from build123d import *

# Parameters (mm, degrees)
BOSS_EXTRUDE1_DEPTH     = 19.05
SKETCH2_R               = 1.26619
CUT_EXTRUDE1_DEPTH      = 18.879441165
CUT_EXTRUDE1_DEPTH_BACK = 28.404441165
SKETCH3_R               = 1.26619
CUT_EXTRUDE2_DEPTH      = 4.175


with BuildPart() as part:
    # Sketch1 → Boss-Extrude1 (new body)
    with BuildSketch(Plane(origin=(0, 0, 0), x_dir=(1, 0, 0), z_dir=(0, 1, 0))):
        Polygon((0, -22.641941165), (0, 22.641941165), (3.175, 22.641941165), (3.175, 4.7625), (21.59, 4.7625), (21.59, 1.5875), (3.175, 1.5875), (3.175, -1.5875), (21.59, -1.5875), (21.59, -4.7625), (3.175, -4.7625), (3.175, -22.641941165), align=None)
    extrude(amount=BOSS_EXTRUDE1_DEPTH)

    # Sketch2 → Cut-Extrude1 (cut, two sides)
    with BuildSketch(Plane.XY.offset(4.7625)) as cut_extrude1_sk:
        with Locations((12.065, 9.525)):
            Circle(SKETCH2_R)
    extrude(amount=CUT_EXTRUDE1_DEPTH, mode=Mode.SUBTRACT)
    extrude(cut_extrude1_sk.sketch, amount=-CUT_EXTRUDE1_DEPTH_BACK, mode=Mode.SUBTRACT)

    # Sketch3 → Cut-Extrude2 (cut, through all)
    with BuildSketch(Plane(origin=(3.175, 0, 0), x_dir=(0, 0, -1), z_dir=(1, 0, 0))):
        with Locations((-15.021941165, 14.9225)):
            Circle(SKETCH3_R)
        with Locations((-15.021941165, 4.1275)):
            Circle(SKETCH3_R)
        with Locations((15.021941165, 4.1275)):
            Circle(SKETCH3_R)
        with Locations((15.021941165, 14.9225)):
            Circle(SKETCH3_R)
    extrude(amount=-CUT_EXTRUDE2_DEPTH, mode=Mode.SUBTRACT)


solid = part.part
Source: CAD feature listing. Evaluate the final solid. Frame: model axes, mm. A direction names the side the tool comes from. Coordinates: 2 decimals unless noted, no trailing zeros. Order: outer loops, then holes, each group sorted by start corner. A loop starts at its lowest first (then second) coordinate and runs counter-clockwise, first axis right, second up. Notation, with made-up numbers: M 76.5,-32 L 126.5,-32 A29 ccw 126.5,-12 Z; hole C -5.75,-22 d10. An arc over 180 degrees is marked long. Write each question's results on one line, items separated by ' | '. Start each with the question number.
Item 1: First-contact query: pin 1 Ø1.5 at (y, z) = (13.5, 7.5) entering from +X (3 decimals); pin 2 Ø4 at (x, y) = (12.065, 9.525) entering from +Z; pin 3 Ø2 at (y, z) = (14.92, -15.02) entering from +X; pin 4 Ø10 at (x, y) = (12, 6.5) entering from -Z. Flat tips, straight axial feed; report the tip coordinate or a pass-through.
Item 2: Cut plane A-A (x = 12). Return loops of the section in (y, z), and give its area (3 significant figures).
Item 3: Line query: probe 1 along Z at (x, y) = (6, 11.5); probe 2 along X at (y, z) = (7.5, -0.5) (3 decimals); probe 3 along Y at (x, z) = (11.25, 4.5). Output: solid intervals per line, ascending.
Item 4: Cut plane D-D (z = -18). Return loops of the section in (x, y) (3 decimals).
Item 5: Draft query along Y for faces 1 (the face through (14, 9, 1.588)), 2 (the face through (1.61, 14.15, -14.02)), 3 (the face through (5, 0, -2)), 4 (the face through (1.61, 4.183, -13.757)). Return one class per face: pulls with the +Y half, pulls with the -Y half, needs draft (parallel to the pull), parting line crosses it, or undercut.
Item 6: Cut plane C-C (y = 15.5). Return loops of the section in (x, z) (1 decimal), and give its area (3 significant figures).
Item 7: Cut plane B-B (x = 8.25). Return loops of the section in (y, z).
Item 8: Set-up query: faces 5 (the face through (10, 9, 4.762)), 6 (the face through (2, 9, 22.642)), 7 (the face through (13.27, 9.91, 3.2)), 8 (the face through (3.175, 9, 0)), 9 (the face through (3.175, 9, -14)). Return all of +Z, -Z, +X, -X, +Y, -Y with unobstructed straight access to the full face (end or side cutting, diameter ignored); none if empty.
Checked values:
1) pin 1: stops at x = 3.175 | pin 2: stops at z = 4.76 | pin 3: passes through | pin 4: stops at z = -4.76
2) outline: M 0,-4.76 L 8.26,-4.76 L 8.26,-1.59 L 0,-1.59 Z; M 0,1.59 L 8.26,1.59 L 8.26,4.76 L 0,4.76 Z; M 10.79,-4.76 L 19.05,-4.76 L 19.05,-1.59 L 10.79,-1.59 Z; M 10.79,1.59 L 19.05,1.59 L 19.05,4.76 L 10.79,4.76 Z | area: 105 mm2
3) probe 1: z = -4.76 to -1.59, 1.59 to 4.76 | probe 2: x = 0 to 3.175 | probe 3: y = 0 to 8.56, 10.49 to 19.05
4) outline: M 0,0 L 3.175,0 L 3.175,19.05 L 0,19.05 Z
5) face 1: needs draft | face 2: undercut | face 3: pulls with the -Y half | face 4: undercut
6) outline: M 0,-22.6 L 3.2,-22.6 L 3.2,-16.1 L 0,-16.1 Z; M 0,-13.9 L 3.2,-13.9 L 3.2,-4.8 L 21.6,-4.8 L 21.6,-1.6 L 3.2,-1.6 L 3.2,1.6 L 21.6,1.6 L 21.6,4.8 L 3.2,4.8 L 3.2,13.9 L 0,13.9 Z; M 0,16.1 L 3.2,16.1 L 3.2,22.6 L 0,22.6 Z | area: 246 mm2
7) outline: M 0,-4.76 L 19.05,-4.76 L 19.05,-1.59 L 0,-1.59 Z; M 0,1.59 L 19.05,1.59 L 19.05,4.76 L 0,4.76 Z
8) face 5: +Z, +X, +Y, -Y | face 6: +Z, +X, -X, +Y, -Y | face 7: +Z, -Z | face 8: +X, +Y, -Y | face 9: -Z, +X, +Y, -Y
